Could you check a few things on this drawing? It's one solid part, dimensions in mm from its lowest x, y, z. Round coordinates to 2 decimals unless told otherwise and drop trailing zeros. Order: outer loops, then holes, each group sorted by start corner. A loop starts at its lowest first (then second) coordinate and runs counter-clockwise, first axis right, second up.
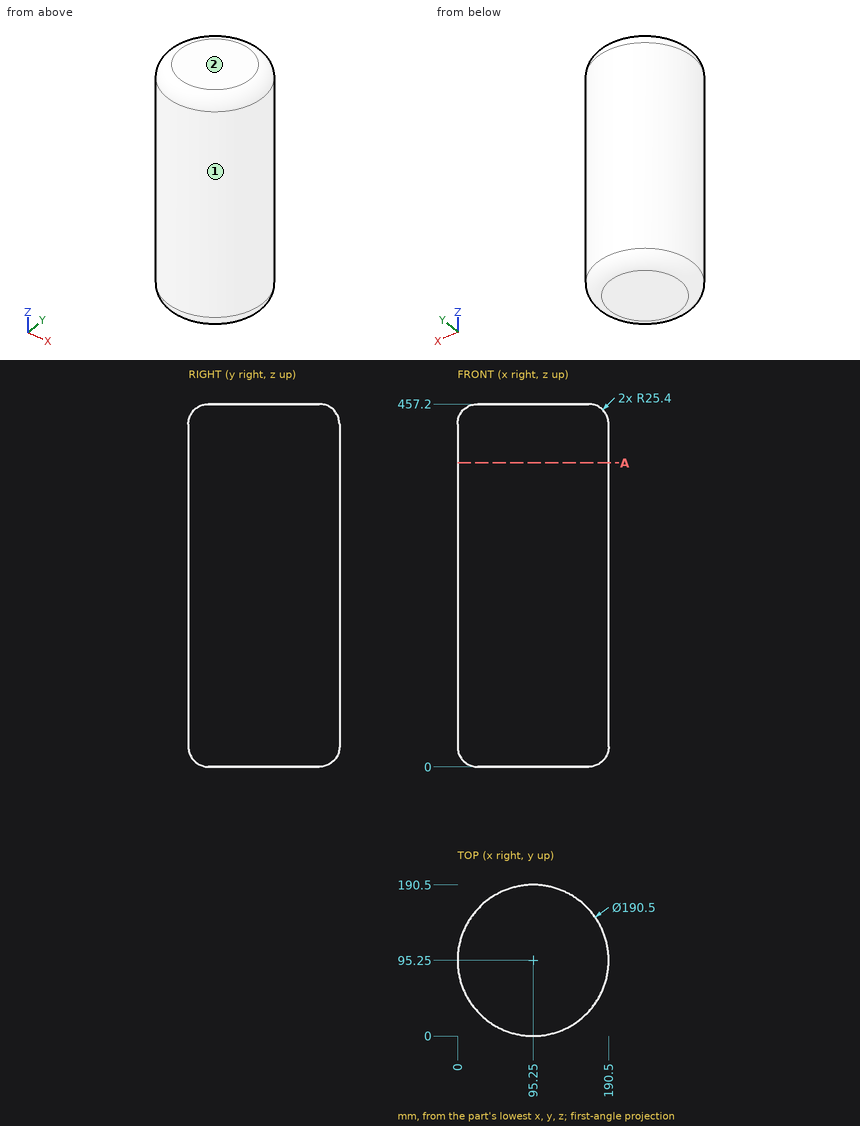
1) I'm going to push flat-ended pins straight in: pin 1 (1 mm diameter, centred on x = 32.5, z = 90.5, fed in from -Y); pin 2 (5 mm diameter, centred on x = 126.5, z = 186.5, fed in from +Y); pin 3 (10 mm diameter, centred on y = 108.5, z = 372, fed in from -X); pin 4 (1 mm diameter, centred on x = 68.5, y = 132.5, fed in from -Z). Where does each tip first touch, or does it pass through?
2) We'd pull the mould along Y, two halves only. Please class the marked faces 1 and 2: +Y half, -Y half, draft (parallel to the pull), parting line (faces both ways), or undercut.
3) If we section it at A-A (z = 383): Write out the boundary of the cut face in (x, y), plus the area to 3 significant figures.
4) I need wall thicknesses on line 1 (X direction, y = 93, z = 192); line 2 (Y direction, x = 92, z = 80.5); line 3 (Z direction, x = 107, y = 177.5). Which ranges of each line are inside material? Lowest first, please.
Solutions:
1. pin 1: stops at y = 23.16
1. pin 2: stops at y = 186.06
1. pin 3: stops at x = 0.36
1. pin 4: stops at z = 0
2. face 1: parting line
2. face 2: draft
3. outline: circle Ø190.5 at (95.25, 95.25)
3. area: 28,500 mm2
4. line 1: x = 0.03 to 190.47
4. line 2: y = 0.06 to 190.44
4. line 3: z = 3.72 to 453.48
